from build123d import *

# Parameters (mm, degrees)
BOSS_EXTRUDE1_DEPTH = 6


with BuildPart() as part:
    # Sketch2 → Boss-Extrude1 (new body)
    with BuildSketch(Plane(origin=(0, 0, 0), x_dir=(1, 0, 0), z_dir=(0, 1, 0))):
        with BuildLine():
            ThreePointArc((1.5, 0), (0, -1.5), (-1.5, 0))
            Line((-1.5, 0), (-3, 0))
            Line((-3, 0), (-3, 5.196152423))
            ThreePointArc((-3, 5.196152423), (-3, -5.196152423), (6, 0))
            ThreePointArc((6, 0), (5.196152423, 3), (3, 5.196152423))
            Line((3, 5.196152423), (3, 0))
            Line((3, 0), (1.5, 0))
        make_face()
        with BuildLine():
            Line((0, 6), (0, 1.5))
            ThreePointArc((0, 1.5), (1.060660172, 1.060660172), (1.5, 0))
            Line((1.5, 0), (3, 0))
            Line((3, 0), (3, 5.196152423))
            ThreePointArc((3, 5.196152423), (1.552914271, 5.795554958), (0, 6))
        make_face()
        with BuildLine():
            ThreePointArc((-1.5, 0), (-1.060660172, 1.060660172), (0, 1.5))
            Line((0, 1.5), (0, 6))
            ThreePointArc((0, 6), (-1.552914271, 5.795554958), (-3, 5.196152423))
            Line((-3, 5.196152423), (-3, 0))
            Line((-3, 0), (-1.5, 0))
        make_face()
        with BuildLine():
            Line((0, 144), (0, 6))
            ThreePointArc((0, 6), (1.552914271, 5.795554958), (3, 5.196152423))
            Line((3, 5.196152423), (3, 144.803847577))
            ThreePointArc((3, 144.803847577), (1.552914271, 144.204445042), (0, 144))
        make_face()
        with BuildLine():
            ThreePointArc((-3, 5.196152423), (-1.552914271, 5.795554958), (0, 6))
            Line((0, 6), (0, 144))
            ThreePointArc((0, 144), (-1.552914271, 144.204445042), (-3, 144.803847577))
            Line((-3, 144.803847577), (-3, 5.196152423))
        make_face()
        with BuildLine():
            Line((0, 148.5), (0, 144))
            ThreePointArc((0, 144), (1.552914271, 144.204445042), (3, 144.803847577))
            Line((3, 144.803847577), (3, 150))
            Line((3, 150), (1.5, 150))
            ThreePointArc((1.5, 150), (1.060660172, 148.939339828), (0, 148.5))
        make_face()
        with BuildLine():
            ThreePointArc((-3, 144.803847577), (-1.552914271, 144.204445042), (0, 144))
            Line((0, 144), (0, 148.5))
            ThreePointArc((0, 148.5), (-1.060660172, 148.939339828), (-1.5, 150))
            Line((-1.5, 150), (-3, 150))
            Line((-3, 150), (-3, 144.803847577))
        make_face()
        with BuildLine():
            ThreePointArc((6, 150), (-3, 155.196152423), (-3, 144.803847577))
            Line((-3, 144.803847577), (-3, 150))
            Line((-3, 150), (-1.5, 150))
            ThreePointArc((-1.5, 150), (0, 151.5), (1.5, 150))
            Line((1.5, 150), (3, 150))
            Line((3, 150), (3, 144.803847577))
            ThreePointArc((3, 144.803847577), (5.196152423, 147), (6, 150))
        make_face()
    extrude(amount=BOSS_EXTRUDE1_DEPTH)


solid = part.part
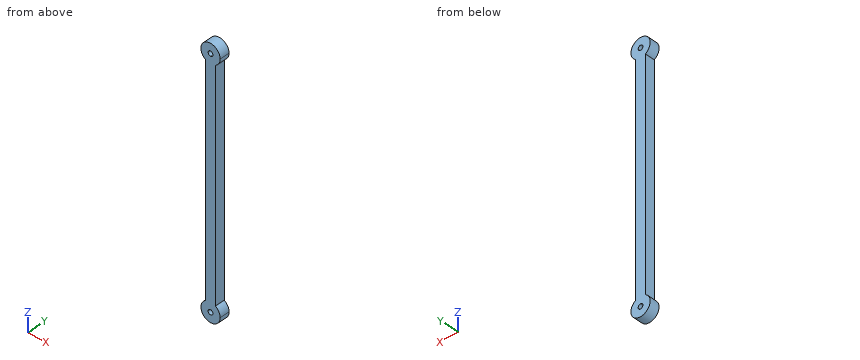
Work out the finished part from the listing and answer in its coordinate system (mm). Give positions to 0.01 mm unless a question says otherwise; leave off trailing zeros. Order: outer loops, then holes, each group sorted by start corner. A loop starts at its lowest first (then second) coordinate and runs counter-clockwise, first axis right, second up. Notation, with made-up numbers: (-22, 36.5) - (30, 36.5) arc R6 cw to (30, 44.5) - close; hole circle Ø10 at (57.25, -12). An arc over 180 degrees is marked (long way). Answer as CSV lines item,"result". Start each with the question number.
Q1. The part is cut by section B-B (z = -127.5). Write down the section's boundary in (x, y), then the cut area to 3 significant figures.
Q2. Given pin 1 Ø1.5 at (y, z) = (0.5, -21) entering from +X; pin 2 Ø2 at (y, z) = (2.5, -86.5) entering from -X; pin 3 Ø3 at (x, y) = (3.5, 1.5) entering from -Z, each flat-ended and moving along its own axis, determine where each tip first touches the part or whether it passes through.
Q3. The part is cut by section A-A (y = 2.05). Write down the section's boundary in (x, z).
Q4. Find the intervals of material crossed by L1, parallel to Z at x = -0.25, y = 3.6; L2, parallel to Z at x = -1, y = 3.4; L3, parallel to Z at x = -5, y = 1.45, in increasing order. Write a range as [from, to].
Check result:
1,outline,"(-3, 0) - (3, 0) - (3, 6) - (-3, 6) - close"
1,area,"36.0 mm²"
2,pin 1,"stops at x = 3"
2,pin 2,"stops at x = -3"
2,pin 3,"stops at z = -155.66"
3,outline,"(-3, -144.8) arc R6 ccw (long way) to (3, -144.8) - (3, -5.2) arc R6 ccw (long way) to (-3, -5.2) - close; hole circle Ø3 at (0, -150); hole circle Ø3 at (0, 0)"
4,L1,"z = [-155.99, -151.48], [-148.52, -1.48], [1.48, 5.99]"
4,L2,"z = [-155.92, -151.12], [-148.88, -1.12], [1.12, 5.92]"
4,L3,"z = [-153.32, -146.68], [-3.32, 3.32]"
